Geometry check sheet. Reference: the model listing, model coordinates, mm. Give positions to 0.01 mm unless a question says otherwise; leave off trailing zeros. Order: outer loops, then holes, each group sorted by start corner. A loop starts at its lowest first (then second) coordinate and runs counter-clockwise, first axis right, second up. Notation, with made-up numbers: M 88.25,-34 L 101.25,-34 A18 cw 101.25,-5 Z; hole C -6.5,13.5 d9. An arc over 180 degrees is marked long. Answer as CSV lines item,"result". Start each with the question number.
Q1. Section check A-A, the plane x = 16.5. Record the boundary of the cut face in (y, z), then the cut area to 3 significant figures.
Q2. Thickness scan on line 1 (Y direction, x = 12.5, z = 11); line 2 (Y direction, x = -17, z = 8); line 3 (Y direction, x = -16.5, z = 4.5). Record the ranges inside material, lowest first.
Q3. Go/stop test with a flat-tipped pin: pin 1 (2.5 mm diameter, centred on x = -16.5, y = 28.5, fed in from -Z). Record where the tip stops, or that it passes through.
Q4. Section check B-B, the plane y = -29.5. Record the boundary of the cut face in (x, z), then the cut area to 3 significant figures.
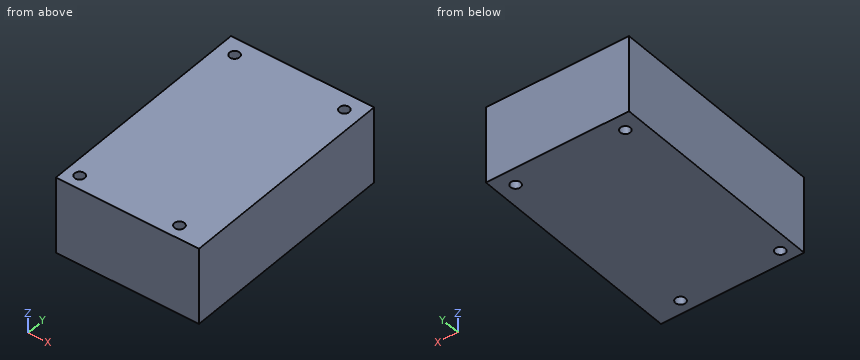
```python
from build123d import *

# Parameters (mm, degrees)
SKETCH1_W           = 67
SKETCH1_H           = 43
BOSS_EXTRUDE1_DEPTH = 23
CUT_EXTRUDE1_REACH  = 47.973
SKETCH2_R           = 1.5


with BuildPart() as part:
    # Sketch1 → Boss-Extrude1 (new body)
    with BuildSketch(Plane(origin=(0, 0, 0), x_dir=(0, 1, 0), z_dir=(0, 0, 1))):
        Rectangle(SKETCH1_W, SKETCH1_H)
    extrude(amount=BOSS_EXTRUDE1_DEPTH)

    # Sketch2 → Cut-Extrude1 (cut, up to next)
    with BuildSketch(Plane.XY.offset(23), mode=Mode.PRIVATE) as cut_extrude1_sk1:
        with Locations((-16.5, 28.5)):
            Circle(SKETCH2_R)
    cut_extrude1_tool1 = extrude(cut_extrude1_sk1.sketch, amount=-CUT_EXTRUDE1_REACH, mode=Mode.PRIVATE) & part.part
    # Sketch2 → Cut-Extrude1 (cut, up to next)
    with BuildSketch(Plane.XY.offset(23), mode=Mode.PRIVATE) as cut_extrude1_sk2:
        with Locations((16.5, 28.5)):
            Circle(SKETCH2_R)
    cut_extrude1_tool2 = extrude(cut_extrude1_sk2.sketch, amount=-CUT_EXTRUDE1_REACH, mode=Mode.PRIVATE) & part.part
    # Sketch2 → Cut-Extrude1 (cut, up to next)
    with BuildSketch(Plane.XY.offset(23), mode=Mode.PRIVATE) as cut_extrude1_sk3:
        with Locations((12.5, -29.5)):
            Circle(SKETCH2_R)
    cut_extrude1_tool3 = extrude(cut_extrude1_sk3.sketch, amount=-CUT_EXTRUDE1_REACH, mode=Mode.PRIVATE) & part.part
    # Sketch2 → Cut-Extrude1 (cut, up to next)
    with BuildSketch(Plane.XY.offset(23), mode=Mode.PRIVATE) as cut_extrude1_sk4:
        with Locations((-17.5, -29.5)):
            Circle(SKETCH2_R)
    cut_extrude1_tool4 = extrude(cut_extrude1_sk4.sketch, amount=-CUT_EXTRUDE1_REACH, mode=Mode.PRIVATE) & part.part
    add(cut_extrude1_tool1.solids().sort_by_distance((-16.5, 28.5, 23))[0], mode=Mode.SUBTRACT)
    add(cut_extrude1_tool2.solids().sort_by_distance((16.5, 28.5, 23))[0], mode=Mode.SUBTRACT)
    add(cut_extrude1_tool3.solids().sort_by_distance((12.5, -29.5, 23))[0], mode=Mode.SUBTRACT)
    add(cut_extrude1_tool4.solids().sort_by_distance((-17.5, -29.5, 23))[0], mode=Mode.SUBTRACT)


solid = part.part
```
Answer block:
1,outline,"M -33.5,0 L 27,0 L 27,23 L -33.5,23 Z; M 30,0 L 33.5,0 L 33.5,23 L 30,23 Z"
1,area,"1,470 mm2"
2,line 1,"y = -33.5 to -31, -28 to 33.5"
2,line 2,"y = -33.5 to -30.91, -28.09 to 27.09, 29.91 to 33.5"
2,line 3,"y = -33.5 to -30.62, -28.38 to 27, 30 to 33.5"
3,pin 1,"passes through"
4,outline,"M -21.5,0 L -19,0 L -19,23 L -21.5,23 Z; M -16,0 L 11,0 L 11,23 L -16,23 Z; M 14,0 L 21.5,0 L 21.5,23 L 14,23 Z"
4,area,"851 mm2"
